The listing builds one solid part. Answer for the finished solid, in the listing's coordinates (mm). A direction names the side the tool comes from. Give positions to 0.01 mm unless a question says otherwise; leave off trailing zeros. Answer in a Markdown table with one row per item. Add a question column.
```python
from build123d import *

# Parameters (mm, degrees)
SALIENTE_EXTRUIR2_DEPTH = 10.5
VACIADO1_T              = -1
CROQUIS4_R              = 20
CROQUIS4_R_2            = 17.5
SALIENTE_EXTRUIR3_DEPTH = 1.5
CROQUIS5_R              = 20
CROQUIS5_R_2            = 17.5
SALIENTE_EXTRUIR4_DEPTH = 0.5
REDONDEO1_R             = 5
REDONDEO2_R             = 0.5
CORTAR_EXTRUIR1_DEPTH   = 53.490475346
CHAFL_N1_SIZE           = 1
CHAFL_N2_SIZE           = 1
CROQUIS7_R              = 0.75
CORTAR_EXTRUIR2_DEPTH   = 1
CROQUIS8_R              = 0.5
CORTAR_EXTRUIR3_DEPTH   = 10
CROQUIS9_R              = 1.25
CORTAR_EXTRUIR4_DEPTH   = 1.5


# Some blends are built 0.0001 mm under size
with BuildPart() as part:
    # Croquis3 → Saliente-Extruir2 (new body)
    with BuildSketch(Plane.XY):
        with BuildLine():
            Line((-16, 23), (16, 23))
            ThreePointArc((16, 23), (20.949747468, 20.949747468), (23, 16))
            Line((23, 16), (23, -16))
            ThreePointArc((23, -16), (20.949747468, -20.949747468), (16, -23))
            Line((16, -23), (-16, -23))
            ThreePointArc((-16, -23), (-20.949747468, -20.949747468), (-23, -16))
            Line((-23, -16), (-23, 16))
            ThreePointArc((-23, 16), (-20.949747468, 20.949747468), (-16, 23))
        make_face()
    extrude(amount=SALIENTE_EXTRUIR2_DEPTH)

    # Vaciado1
    vaciado1_openings = [part.faces().sort_by_distance(p)[0] for p in [
        (0, 0, 10.5),
    ]]
    offset(amount=VACIADO1_T, openings=vaciado1_openings, kind=Kind.INTERSECTION)



with BuildPart() as body_2:
    # Croquis4 → Saliente-Extruir3 (new body)
    # profile 1 of 2: a face of its own
    with BuildSketch(Plane.XY.offset(6.25)):
        with BuildLine():
            Line((22, -16), (22, 16))
            ThreePointArc((22, 16), (20.242640687, 20.242640687), (16, 22))
            Line((16, 22), (-16, 22))
            ThreePointArc((-16, 22), (-20.242640687, 20.242640687), (-22, 16))
            Line((-22, 16), (-22, -16))
            ThreePointArc((-22, -16), (-20.242640687, -20.242640687), (-16, -22))
            Line((-16, -22), (16, -22))
            ThreePointArc((16, -22), (20.242640687, -20.242640687), (22, -16))
        make_face()
        Circle(CROQUIS4_R, mode=Mode.SUBTRACT)
    # profile 2 of 2: a face of its own
    with BuildSketch(Plane.XY.offset(6.25)):
        Circle(CROQUIS4_R)
        Circle(CROQUIS4_R_2, mode=Mode.SUBTRACT)
    extrude(amount=SALIENTE_EXTRUIR3_DEPTH)


with BuildPart() as part_1:
    add(part.part)

    add(body_2.part)  # Saliente-Extruir4 merges body 2
    # Croquis5 → Saliente-Extruir4 (add)
    with BuildSketch(Plane.XY.offset(7.75)):
        Circle(CROQUIS5_R)
        Circle(CROQUIS5_R_2, mode=Mode.SUBTRACT)
    extrude(amount=SALIENTE_EXTRUIR4_DEPTH)

    # Redondeo1
    # the kernel refuses this fillet: 5 mm, written as the material it adds along each edge
    with BuildSketch(Plane(origin=(0, 0, 7.75), x_dir=(1, 0, 0), z_dir=(0, -1, 0))) as redondeo1_piece_1:
        with BuildLine():
            CenterArc((22.179449472, 5), REDONDEO1_R, 244.158067237, 25.841932763)
            Line((22.179449472, 0), (22.179449472, -0.1))
            Line((22.179449472, -0.1), (20, -0.1))
            Line((20, -0.1), (19.9, 0))
            ThreePointArc((19.9, 0), (19.9, 0.25), (19.956411011, 0.41))
            Line((19.956411011, 0.41), (20, 0.5))
        make_face()
    revolve(axis=Axis((0, 0, 7.75), (0, 0, 1)))

    # Redondeo2
    redondeo2_edges = [part_1.edges().sort_by_distance(p)[0] for p in [
        (-17.5, 0, 6.25),
        (-17.5, 0, 8.25),
    ]]
    fillet(redondeo2_edges, radius=REDONDEO2_R)

    # Croquis6 → Cortar-Extruir1 (cut, through all)
    with BuildSketch(Plane.ZY.offset(23)):
        with BuildLine():
            Line((1.625, -13), (1.625, 13))
            ThreePointArc((1.625, 13), (3.125, 14.5), (4.625, 13))
            Line((4.625, 13), (4.625, -13))
            ThreePointArc((4.625, -13), (3.125, -14.5), (1.625, -13))
        make_face()
    extrude(amount=-CORTAR_EXTRUIR1_DEPTH, mode=Mode.SUBTRACT)

    # Chaflán1
    chafl_n1_edges = [part_1.edges().sort_by_distance(p)[0] for p in [
        (-20.949747468, 20.949747468, 10.5),
        (-23, 0, 10.5),
        (-20.949747468, -20.949747468, 10.5),
        (0, -23, 10.5),
        (20.949747468, -20.949747468, 10.5),
        (23, 0, 10.5),
        (20.949747468, 20.949747468, 10.5),
        (0, 23, 10.5),
    ]]
    chamfer(chafl_n1_edges, length=CHAFL_N1_SIZE - 0.0001)  # a hair under: the kernel refuses the full size

    # Chaflán2
    chafl_n2_edges = [part_1.edges().sort_by_distance(p)[0] for p in [
        (0, 23, 0),
        (20.949747468, 20.949747468, 0),
        (23, 0, 0),
        (20.949747468, -20.949747468, 0),
        (0, -23, 0),
        (-20.949747468, -20.949747468, 0),
        (-23, 0, 0),
        (-20.949747468, 20.949747468, 0),
    ]]
    chamfer(chafl_n2_edges, length=CHAFL_N2_SIZE)

    # Croquis7 → Cortar-Extruir2 (cut)
    with BuildSketch(Plane(origin=(0, 0, 0), x_dir=(-1, 0, 0), z_dir=(0, 0, -1))):
        with Locations((-19, 9)):
            Circle(CROQUIS7_R)
        with Locations(Location((-19, -9, 0), (0, 0, 180))):
            Circle(CROQUIS7_R)
        with Locations((19, -9)):
            Circle(CROQUIS7_R)
        with Locations(Location((19, 9, 0), (0, 0, 180))):
            Circle(CROQUIS7_R)
    extrude(amount=-CORTAR_EXTRUIR2_DEPTH, mode=Mode.SUBTRACT)

    # Croquis8 → Cortar-Extruir3 (cut)
    with BuildSketch(Plane.XZ.offset(23)):
        with Locations(Location((0, 5.25, 0), (0, 0, 270))):
            Circle(CROQUIS8_R)
    extrude(amount=-CORTAR_EXTRUIR3_DEPTH, mode=Mode.SUBTRACT)

    # Croquis9 → Cortar-Extruir4 (cut)
    with BuildSketch(Plane.XY.offset(7.75)):
        with Locations((18.3, 18.3)):
            Circle(CROQUIS9_R)
        with Locations(Location((-18.3, 18.3, 0), (0, 0, 180))):
            Circle(CROQUIS9_R)
        with Locations((-18.3, -18.3)):
            Circle(CROQUIS9_R)
        with Locations(Location((18.3, -18.3, 0), (0, 0, 180))):
            Circle(CROQUIS9_R)
    extrude(amount=-CORTAR_EXTRUIR4_DEPTH, mode=Mode.SUBTRACT)


solid = part_1.part
```
(1) Straight lines are drawn through the part: line 1 (Y direction, x = -9.5, z = 1.5); line 2 (Z direction, x = -18.5, y = -4). For each, find the intervals that lie inside material, in ascending order.
(2) Find section A-A, the plane x = -19. Give the number of separate pieces and of enclosed holes in the cut face, plus the area to 3 significant figures.
(3) Each of these flat-tipped pins is pushed along its axis until it touches: P1, Ø12, axis at x = -9, y = 1.5, coming from the +Z side; P2, Ø0.8, axis at x = 22.5, y = 1.5, coming from the +Z side; P3, Ø9.5, axis at x = 13.5, y = 8, coming from the +Z side. Where does it stop, or does it pass through?
(4) For faces 1 (the face through (22.5, 0.2, 10)), 2 (the face through (22.5, -0.2, 1.625)), 3 (the face through (20.289, -20.196, 3.588)), 4 (the face through (17.723, -17.191, 7.01)), determine the directions among +Z, -Z, +X, -X, +Y, -Y from which every point of the face is accessible in a straight line to the end or side of a thin tool.
(5) The mould has two halves that part along Y. Classify faces 5 (the face through (-23, 0, 6)), 6 (the face through (0, 22, 9)), 7 (the face through (-20.413, 20.317, 10.326)), 8 (the face through (17, 17, 7.75)): +Y half, -Y half, draft (parallel to the pull), parting line (faces both ways), or undercut.
Answer key:
| question | item | result |
|---|---|---|
| 1 | line 1 | -23 to -22, 22 to 23 |
| 1 | line 2 | 0 to 1, 6.25 to 8.25 |
| 2 | separate pieces | 4 |
| 2 | enclosed holes | 0 |
| 2 | area | 126 mm² |
| 3 | P1 | z = 1 |
| 3 | P2 | z = 10.4 |
| 3 | P3 | z = 8.25 |
| 4 | face 1 | +Z, +X, +Y, -Y |
| 4 | face 2 | +X, -X |
| 4 | face 3 | none |
| 4 | face 4 | +Z |
| 5 | face 5 | draft |
| 5 | face 6 | undercut |
| 5 | face 7 | +Y half |
| 5 | face 8 | undercut |
